Build history of the part. All positions in model axes, mm. A direction names the side the tool comes from. Give positions to 0.01 mm unless a question says otherwise; leave off trailing zeros. Write each loop counter-clockwise with the first axis right and the second up, starting at its lowest first coordinate (ties: lowest second). Pieces come first, ordered by that corner, then holes. Notation, with made-up numbers: M -20.75,60.5 L 14.25,60.5 A18 cw 14.25,66.5 Z; hole C -5,10.5 d6. An arc over 180 degrees is marked long. One line per item, written item: value. Start each with the question number.
Autodesk Inventor part; units mm, degrees
ref_plane "YZ Plane" through (0, 0, 0) normal (1, 0, 0) x (0, 1, 0)
ref_plane "XZ Plane" through (0, 0, 0) normal (0, 1, 0) x (-1, 0, 0)
ref_plane "XY Plane" through (0, 0, 0) normal (0, 0, 1) x (1, 0, 0)
sketch "Sketch1" plane through (0, 0, 0) normal (1, 0, 0) x (0, 1, 0)
  line L0 (-27.5, 22.5) -> (27.5, 22.5)
  line L1 (27.5, 22.5) -> (27.5, -22.5)
  line L2 (27.5, -22.5) -> (-27.5, -22.5)
  line L3 (-27.5, -22.5) -> (-27.5, 22.5)
  line L4 (-27.5, 22.5) -> (27.5, -22.5) construction
  line L5 (27.5, 22.5) -> (-27.5, -22.5) construction
  line L6 (32.5, 37.5) -> (-32.5, 37.5)
  line L7 (-32.5, 37.5) -> (-32.5, -162.5)
  line L8 (-32.5, -162.5) -> (32.5, -162.5)
  line L9 (32.5, -162.5) -> (32.5, 37.5)
  line L10 (0, 0) -> (0, -107.0279) construction
  dimension "d0" = 45
  dimension "d1" = 55
  dimension "d2" = 65
  dimension "d3" = 200
  dimension "d4" = 15
extrude "Extrusion1" add sketch "Sketch1" along normal mid plane 10 contours L0 L1 L2 L3 | L9 L8 L7 L6
hole "Hole1" at (0, 27.5, 22.5) at (0, -27.5, 22.5) at (0, -27.5, -22.5) at (0, 27.5, -22.5) direction (-1, 0, 0) diameter 4.2 end through all both
sketch "Sketch3" plane through (5, 0, 0) normal (1, 0, 0) x (0, 0, -1)
  circle A0 centre (22.5, -27.5) radius 2.1
  circle A1 centre (-22.5, 27.5) radius 2.1
  circle A2 centre (-22.5, -27.5) radius 2.1
  circle A3 centre (22.5, 27.5) radius 2.1
  line L0 (-37.5, -32.5) -> (162.5, -32.5)
  line L1 (162.5, -32.5) -> (162.5, 32.5)
  line L2 (162.5, 32.5) -> (-37.5, 32.5)
  line L3 (-37.5, 32.5) -> (-37.5, -32.5)
  line L4 (162.5, 0) -> (-37.5, 0) construction
  line L5 (-37.5, 32.5) -> (-37.5, -32.5)
  line L6 (162.5, -32.5) -> (162.5, 32.5)
  arc A4 (159.6938, 40) -> (159.6938, -40) centre (172.5, 0) ccw construction
  arc A5 (153.5955, 59.0476) -> (153.5955, -59.0476) centre (172.5, 0) ccw
  arc A6 (165.792, 20.9524) -> (165.792, -20.9524) centre (172.5, 0) ccw
  arc A7 (165.792, 20.9524) -> (153.5955, 59.0476) centre (159.6938, 40) ccw
  arc A8 (153.5955, -59.0476) -> (165.792, -20.9524) centre (159.6938, -40) ccw
  arc A9 (157.4984, 46.8571) -> (157.4984, -46.8571) centre (172.5, 0) ccw
  arc A10 (157.4984, -46.8571) -> (161.8891, -33.1429) centre (159.6938, -40) ccw
  arc A11 (161.8891, 33.1429) -> (161.8891, -33.1429) centre (172.5, 0) ccw
  arc A12 (161.8891, 33.1429) -> (157.4984, 46.8571) centre (159.6938, 40) ccw
  circle A13 centre (130.5, 0) radius 7.2
  point P0 (0, 0)
  point P1 (162.5, 0)
  point P2 (135.5623, -32.5)
  point P3 (119.7009, -32.5)
  point P4 (113.3868, -25)
  point P5 (160.0585, -32.5)
  point P6 (160.0585, 32.5)
  point P7 (113.3868, 25)
  point P8 (119.7009, 32.5)
  point P9 (135.5623, 32.5)
  point P10 (116.802, 25)
  point P11 (116.802, -25)
  point P12 (123.3, 0)
  point P13 (137.7, 0)
  point P14 (162.5, -19.5959)
  point P15 (162.5, 19.5959)
  dimension "d27" = 42
  dimension "d28" = 20
  dimension "d29" = 10
  dimension "d30" = 80
  dimension "d32" = 7.2
extrude "Extrusion2" add sketch "Sketch3" against normal blind 10 contours A5 L2 A9 L0 | L0 A9 A10 A11 L1 A6 A8 A5 | A9 A13 A11 L0 | L0 A11 A10 A9 | A5 A7 A6 L1 L2 A11 A12 A9 | A11 L2 L1 A6 L0 | A9 L2 A11 A13 | A13 | A9 A12 A11 L2
extrude "Extrusion3" cut sketch "Sketch3" against normal blind 85 contours A9 L2 A11 A13 | A13 | A9 A12 A11 L2
extrude "Extrusion4" cut sketch "Sketch3" against normal blind 85 contours A6 L1
chamfer "Chamfer1" distance 24 angle 45 2 edges at (0, 32.5, -119.7009) (0, -32.5, -119.7009)
fillet "Fillet1" radius 119 2 edges at (0, 32.5, -95.7009) (0, -32.5, -95.7009)
sketch "Sketch4" plane through (5, 0, 0) normal (1, 0, 0) x (0, 0, -1)
  arc A0 (118.4927, -42.4637) -> (70.8263, -32.5) centre (70.8263, -151.5) ccw
  line L0 (70.8263, -32.5) -> (178.2342, -32.5)
  arc A1 (153.5955, -59.0476) -> (165.792, -20.9524) centre (159.6938, -40) ccw
  arc A2 (135.9994, -50.1169) -> (153.5955, -59.0476) centre (172.5, 0) ccw
  line L1 (135.9994, -50.1169) -> (118.4927, -42.4637)
  point P0 (0, 0)
extrude "Extrusion5" cut sketch "Sketch4" against normal blind 36.25
fillet "Fillet2" radius 2 1 edges at (0, -32.5, -178.2342)
sketch "Sketch5" plane through (5, 0, 0) normal (1, 0, 0) x (0, 0, -1)
  line L0 (0, 0) -> (0, 9.6714)
  line L1 (-5, 0) -> (5, 0)
  dimension "d46" = 10
hole "Hole3" at (5, 0, -5) at (5, 0, 5) direction (-1, 0, 0) diameter 1.8 end through all
sketch "Sketch6" plane through (5, 0, 0) normal (1, 0, 0) x (0, 0, -1)
  circle A0 centre (5, 0) radius 0.9
  circle A1 centre (-5, 0) radius 0.9
  arc A2 (174.9826, -32.5) -> (176.6814, -29.4444) centre (174.9826, -30.5) ccw
  arc A3 (176.6814, -29.4444) -> (165.792, -20.9524) centre (159.6938, -40) ccw
  arc A4 (165.792, 20.9524) -> (165.792, -20.9524) centre (172.5, 0) ccw
  arc A5 (165.792, 20.9524) -> (153.5955, 59.0476) centre (159.6938, 40) ccw
  arc A6 (153.5955, 59.0476) -> (135.9994, 50.1169) centre (172.5, 0) ccw
  line L0 (118.4927, 42.4637) -> (135.9994, 50.1169)
  arc A7 (70.8263, 32.5) -> (118.4927, 42.4637) centre (70.8263, 151.5) ccw
  line L1 (70.8263, 32.5) -> (-37.5, 32.5)
  line L2 (-37.5, 32.5) -> (-37.5, -32.5)
  line L3 (-37.5, -32.5) -> (174.9826, -32.5)
  circle A8 centre (22.5, 27.5) radius 2.1
  circle A9 centre (-22.5, -27.5) radius 2.1
  circle A10 centre (-22.5, 27.5) radius 2.1
  circle A11 centre (22.5, -27.5) radius 2.1
  arc A12 (123.3, 0) -> (137.7, 0) centre (130.5, 0) ccw
  arc A13 (157.4984, 46.8571) -> (123.3, 0) centre (172.5, 0) ccw
  arc A14 (161.8891, 33.1429) -> (157.4984, 46.8571) centre (159.6938, 40) ccw
  arc A15 (161.8891, 33.1429) -> (137.7, 0) centre (172.5, 0) ccw
  line L4 (-37.5, 32.5) -> (70.8263, 32.5)
  line L5 (70.8263, 32.5) -> (70.8263, -32.5) construction
  line L6 (174.9826, -32.5) -> (-37.5, -32.5)
  line L7 (43.3263, 32.5) -> (98.3263, 32.5) construction
  line L8 (70.8263, 32.5) -> (-37.5, 32.5)
  line L9 (43.3263, 22.5) -> (98.3263, 22.5)
  line L10 (98.3263, 42.5) -> (43.3263, 42.5)
  arc A16 (43.3263, 42.5) -> (43.3263, 22.5) centre (43.3263, 32.5) ccw
  arc A17 (98.3263, 22.5) -> (98.3263, 42.5) centre (98.3263, 32.5) ccw
  line L11 (70.8263, 0) -> (130.5, 0) construction
  line L12 (43.3263, -22.5) -> (98.3263, -22.5)
  line L13 (98.3263, -42.5) -> (43.3263, -42.5)
  arc A18 (43.3263, -22.5) -> (43.3263, -42.5) centre (43.3263, -32.5) ccw
  arc A19 (98.3263, -42.5) -> (98.3263, -22.5) centre (98.3263, -32.5) ccw
  point P0 (0, 0)
  point P1 (106.6621, 38.024)
  point P2 (33.3263, 32.5)
  dimension "d57" = 10
  dimension "d58" = 55
extrude "Extrusion6" cut sketch "Sketch6" against normal blind 27.5 contours A19 L13 A18 L3 | L3 A18 L12 A19 | L1 A7 A17 L9 A16
chamfer "Chamfer2" distance 8.5 angle 45 2 edges at (0, -32.5, -108.3263) (0, 38.024, -106.6621)
chamfer "Chamfer3" distance 5.75 angle 45 2 edges at (0, -32.5, -33.3263) (0, 32.5, -33.3263)
fillet "Fillet3" radius 6.5 1 edges at (0, -32.5, 37.5)
properties part number "16_Khau_hai" material "Stainless Steel, Austenitic"
1) Mould opens along Y. For faces 4 (the face through (-0.07, -28.131, 20.497)), 5 (the face through (0.07, -7.2, -130.34)), 6 (the face through (0.07, -23.11, -101.77)), 7 (the face through (0, 32.5, 5)) say: released by +Y, released by -Y, zero draft, split by the parting line, or undercut.
2) Drop flat-ended pins along their axis: P1, Ø1.4, axis at y = 0, z = -5, coming from the +X side; P2, Ø3, axis at x = 0.5, y = -12.5, coming from the -Z side; P3, Ø5, axis at x = -2.5, z = 7.5, coming from the +Y side; P4, Ø2, axis at x = -3.5, y = 13.5, coming from the -Z side. Give the stop position or say it passes through.
3) Tool access for faces 1 (the face through (-0.07, -28.6, -110.69)), 2 (the face through (0.1, 20.8, -144.6)), 3 (the face through (0.07, 23.728, -38.526)): list every direction of +Z, -Z, +X, -X, +Y, -Y with a clear straight run to the whole face (end or side of a thin tool).
4) Band-saw the part on C-C (y = -13). List the corners of the cut face in (x, z), then the cut area to 3 significant figures.
5) Probe line 1 along Y through (x, z) = (1.25, 22.5); line 2 along Y through (x, z) = (1.75, -5); line 3 along Y through (x, z) = (0.25, 21). List the from-to ranges inside material, lowest first. Write a range as from..to.
6) Band-saw the part on B-B (z = -59). List the corners of the cut face in (x, y), then the cut area to 3 significant figures.
7) Band-saw the part on D-D (x = -1.5). Count the separate pieces of the cut face and the enclosed holes in it, then the cut area to 3 significant figures.
8) Band-saw the part on A-A (z = -22.5). List the corners of the cut face in (x, y), then the cut area to 3 significant figures.
Model answer:
1. face 4: undercut
1. face 5: undercut
1. face 6: released by -Y
1. face 7: released by +Y
2. P1: passes through
2. P2: stops at z = -155.53
2. P3: stops at y = 32.5
2. P4: stops at z = -155.95
3. face 1: +X, -X, -Y
3. face 2: +X, -X
3. face 3: +X, -X, +Y
4. outline: M -5,-154.75 L 5,-154.75 L 5,37.5 L -5,37.5 Z
4. area: 1,920 mm²
5. line 1: y = -32.5..-29.6, -25.4..25.4, 29.6..32.5
5. line 2: y = -32.5..-0.9, 0.9..32.5
5. line 3: y = -32.5..-28.97, -26.03..26.03, 28.97..32.5
6. outline: M -5,-22.5 L 5,-22.5 L 5,22.5 L -5,22.5 Z
6. area: 450 mm²
7. separate pieces: 1
7. enclosed holes: 7
7. area: 11,800 mm²
8. outline: M -5,-32.5 L 5,-32.5 L 5,-29.6 L -5,-29.6 Z; M -5,-25.4 L 5,-25.4 L 5,25.4 L -5,25.4 Z; M -5,29.6 L 5,29.6 L 5,32.5 L -5,32.5 Z
8. area: 566 mm²
